The listing builds one solid part. Answer for the finished solid, in the listing's coordinates (mm). Face numbers are marked on the shaded views. A direction names the side the tool comes from. Coordinates: 2 decimals unless noted, no trailing zeros. Order: outer loops, then holes, each group sorted by start corner. A loop starts at its lowest first (then second) coordinate and runs counter-clockwise, first axis right, second up. Notation, with made-up numbers: (49.25, -23) -> (106.25, -23) arc R5 cw to (106.25, -18) -> close; hole circle Ø9 at (20, 79.5). An arc over 180 degrees is marked (long way). Answer in a Markdown table with one row per item.
```python
from build123d import *

# Parameters (mm, degrees)
SKETCH2_W           = 30
SKETCH2_H           = 35
BOSS_EXTRUDE1_DEPTH = 3
FILLET1_R           = 5
SKETCH3_R           = 2
CUT_EXTRUDE1_DEPTH  = 10
SKETCH6_R           = 4
BOSS_EXTRUDE2_DEPTH = 45
FILLET2_R           = 1


with BuildPart() as part:
    # Sketch2 → Boss-Extrude1 (new body)
    with BuildSketch(Plane.XY):
        with Locations((15, -17.5)):
            Rectangle(SKETCH2_W, SKETCH2_H)
    extrude(amount=BOSS_EXTRUDE1_DEPTH)

    # Fillet1
    fillet1_edges = [part.edges().sort_by_distance(p)[0] for p in [
        (0, 0, 1.5),
        (30, 0, 1.5),
        (30, -35, 1.5),
        (0, -35, 1.5),
    ]]
    fillet(fillet1_edges, radius=FILLET1_R)

    # Sketch3 → Cut-Extrude1 (cut)
    with BuildSketch(Plane.XY.offset(3)):
        with Locations((6, -5.5)):
            Circle(SKETCH3_R)
        with Locations((24, -5.5)):
            Circle(SKETCH3_R)
        with Locations((6, -29.5)):
            Circle(SKETCH3_R)
        with Locations((24, -29.5)):
            Circle(SKETCH3_R)
    extrude(amount=-CUT_EXTRUDE1_DEPTH, mode=Mode.SUBTRACT)

    # Sketch6 → Boss-Extrude2 (add)
    with BuildSketch(Plane(origin=(0, 0, 0), x_dir=(-1, 0, 0), z_dir=(0, 0, -1))):
        with Locations(Location((-15, -17.5, 0), (0, 0, 180))):
            Circle(SKETCH6_R)
    extrude(amount=BOSS_EXTRUDE2_DEPTH)

    # Fillet2
    fillet2_edges = [part.edges().sort_by_distance(p)[0] for p in [
        (11, -17.5, -45),
    ]]
    fillet(fillet2_edges, radius=FILLET2_R)


solid = part.part
```
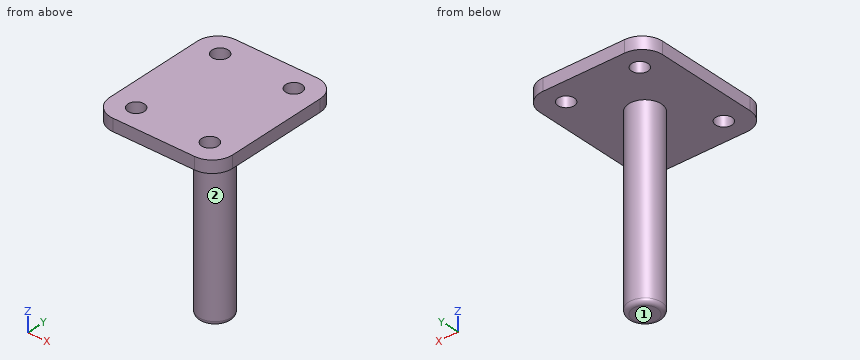
(1) Which of the six approach directions +Z, -Z, +X, -X, +Y, -Y give full straight-line access (tool end or side, diameter ignored) to the marked faces 1 and 2?
Check values:
| item | result |
|---|---|
| face 1 | -Z, +X, -X, +Y, -Y |
| face 2 | -Z |
(2) Flat-ended cylindrical pins translate along their axes: pin 1 (12 mm diameter, centred on y = -19.5, z = -21.5, fed in from -X); pin 2 (10 mm diameter, centred on x = 17.5, y = -28, fed in from -Z); pin 3 (12 mm diameter, centred on x = 9.5, z = -17, fed in from +Y). Find the tip coordinate at first contact, or state that the pin passes through.
Check values:
| item | result |
|---|---|
| pin 1 | x = 11 |
| pin 2 | z = 0 |
| pin 3 | y = -13.5 |
(3) A cutting plane is placed at C-C, the plane z = -14.5. Determine the outline of the cut face in (x, y).
Check values:
| item | result |
|---|---|
| outline | circle Ø8 at (15, -17.5) |
(4) A cutting plane is placed at D-D, the plane x = 15. Determine the outline of the cut face in (y, z).
Check values:
| item | result |
|---|---|
| outline | (-35, 0) -> (-21.5, 0) -> (-21.5, -44) arc R1 ccw to (-20.5, -45) -> (-14.5, -45) arc R1 ccw to (-13.5, -44) -> (-13.5, 0) -> (0, 0) -> (0, 3) -> (-35, 3) -> close |
(5) A cutting plane is placed at B-B, the plane y = -17.5. Determine the outline of the cut face in (x, z), then the cut area to 3 significant figures.
Check values:
| item | result |
|---|---|
| outline | (0, 0) -> (11, 0) -> (11, -44) arc R1 ccw to (12, -45) -> (18, -45) arc R1 ccw to (19, -44) -> (19, 0) -> (30, 0) -> (30, 3) -> (0, 3) -> close |
| area | 450 mm² |
(6) A cutting plane is placed at A-A, the plane x = 24. Determine the outline of the cut face in (y, z).
Check values:
| item | result |
|---|---|
| outline | (-35, 0) -> (-31.5, 0) -> (-31.5, 3) -> (-35, 3) -> close; (-27.5, 0) -> (-7.5, 0) -> (-7.5, 3) -> (-27.5, 3) -> close; (-3.5, 0) -> (0, 0) -> (0, 3) -> (-3.5, 3) -> close |
(7) Find the intervals of material crossed by line 1 along Y through (x, z) = (6, 1.85); line 2 along Z through (x, y) = (24, -27); line 3 along X through (y, z) = (-29, 1), in increasing order. Write a range as from..to.
Check values:
| item | result |
|---|---|
| line 1 | -35..-31.5, -27.5..-7.5, -3.5..0 |
| line 2 | 0..3 |
| line 3 | 0..4.06, 7.94..22.06, 25.94..30 |
